Geometry check sheet. Reference: the model listing, model coordinates, mm. Round coordinates to 2 decimals unless told otherwise and drop trailing zeros. Write each loop counter-clockwise with the first axis right and the second up, starting at its lowest first coordinate (ties: lowest second). Pieces come first, ordered by that corner, then holes. Notation, with made-up numbers: (-31, 24) -> (10, 24) arc R18 ccw to (10, 30) -> close; hole circle Ø11 at (65.25, 56.25). An arc over 180 degrees is marked (long way). One line per question, with ' | ' between items.
```python
from build123d import *

# Parameters (mm, degrees)
F1_DEPTH  = 38.1
F2_R      = 9.3756609964
F3_DEPTH  = 50.8
F5_DEPTH  = 76.2
F7_DEPTH  = 76.2
F9_DEPTH  = 76.2
F11_DEPTH = 76.2
F13_DEPTH = 76.2
F14_R     = 1.8366933485
F16_DEPTH = 76.2
F15_R     = 1.8367030573
F17_DEPTH = 76.2


with BuildPart() as f1:
    # F0 (on Front) → F1 (new body)
    with BuildSketch(Plane.XZ):
        Polygon((0, 63.5), (0, 0), (302.4093748547, 0), (302.4093748547, 25.4), align=None)
    extrude(amount=F1_DEPTH)

    # F2 (on face) → F3 (cut)
    with BuildSketch(Plane(origin=(0, 0, 0), x_dir=(0, -1, 0), z_dir=(-1, 0, 0))):
        with Locations((19.05, 31.75)):
            Circle(F2_R)
    extrude(amount=-F3_DEPTH, mode=Mode.SUBTRACT)

    # F4 (on face) → F5 (cut)
    with BuildSketch(Plane.XZ.offset(38.1)):
        with BuildLine():
            Line((269.3568159992, 29.5642309965), (61.5471690917, 55.7457855564))
            add(Edge.make_bspline(
                [(61.5471690917, 55.7457855564), (58.8507788185, 47.0996876999), (48.0888197805, 12.590977334), (174.5673004743, 22.2930190768), (269.3568159992, 29.5642309965)],
                knots=[0, 0, 0, 0, 0.2505482751, 1, 1, 1, 1], degree=3))
        make_face()
    extrude(amount=-F5_DEPTH, mode=Mode.SUBTRACT)

    # F6 (on face) → F7 (cut)
    with BuildSketch(Plane.XZ.offset(38.1)):
        with BuildLine():
            Line((0, 63.5), (0, 49.8412624001))
            Line((0, 49.8412624001), (59.7987414655, 49.8412624001))
            add(Edge.make_bspline(
                [(61.5471690917, 55.7457855564), (60.9299090319, 53.7665131444), (60.3126489722, 51.7872407325), (59.7987414655, 49.8412624001)],
                knots=[0, 0, 0, 0, 0.057355734, 0.057355734, 0.057355734, 0.057355734], degree=3))
            Line((61.5471690917, 55.7457855564), (0, 63.5))
        make_face()
    extrude(amount=-F7_DEPTH, mode=Mode.SUBTRACT)

    # F8 (on face) → F9 (cut)
    with BuildSketch(Plane.XZ.offset(38.1)):
        with BuildLine():
            Line((59.7987414655, 49.8412624001), (52.5512769818, 49.8412624001))
            Line((52.5512769818, 49.8412624001), (59.7987414652, 35.7225287025))
            add(Edge.make_bspline(
                [(59.7987414655, 49.8412624001), (58.4403182232, 44.6974142144), (57.8040351338, 39.7861968724), (59.7987414652, 35.7225287025)],
                knots=[0.057355734, 0.057355734, 0.057355734, 0.057355734, 0.2089654324, 0.2089654324, 0.2089654324, 0.2089654324], degree=3))
        make_face()
    extrude(amount=-F9_DEPTH, mode=Mode.SUBTRACT)

    # F10 (on face) → F11 (cut)
    with BuildSketch(Plane.XZ.offset(38.1)):
        Polygon((302.4093748547, 25.4), (269.3568159992, 29.5642309965), (302.4093748547, 6.536568515), align=None)
    extrude(amount=-F11_DEPTH, mode=Mode.SUBTRACT)

    # F12 (on face) → F13 (cut)
    with BuildSketch(Plane.XZ.offset(38.1)):
        with BuildLine():
            add(Edge.make_bspline(
                [(240.1607868718, 27.3452845776), (249.8366976467, 28.0668616255), (259.596756823, 28.815546311), (269.3568159992, 29.5642309965)],
                knots=[0.9228322548, 0.9228322548, 0.9228322548, 0.9228322548, 1, 1, 1, 1], degree=3))
            Line((240.1607868718, 27.3452845776), (302.4093748547, 6.536568515))
            Line((302.4093748547, 6.536568515), (269.3568159992, 29.5642309965))
        make_face()
    extrude(amount=-F13_DEPTH, mode=Mode.SUBTRACT)

    # F14 (on face) → F16 (cut)
    with BuildSketch(Plane.XZ.offset(38.1)):
        with Locations((6.889551878, 5.4092812352)):
            Circle(F14_R)
    extrude(amount=-F16_DEPTH, mode=Mode.SUBTRACT)

    # F15 (on face) → F17 (cut)
    with BuildSketch(Plane.XZ.offset(38.1)):
        with Locations((292.2985553741, 3.6882217973)):
            Circle(F15_R)
    extrude(amount=-F17_DEPTH, mode=Mode.SUBTRACT)


solid = f1.part
```
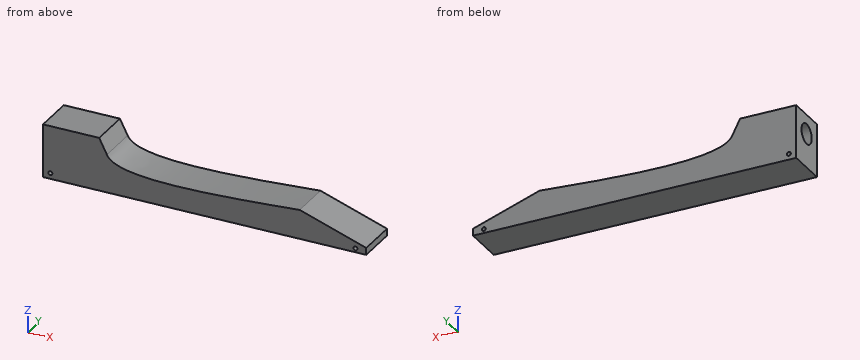
(1) Sectioned sample at B-B on y = -24. Count the separate pieces of the cut face and the enclosed holes in it, then the cut area to 3 significant figures.
Resolved:
separate pieces: 1 | enclosed holes: 2 | area: 7,500 mm2
(2) Sectioned sample at C-C on x = 259.5. Record the cut outline in (y, z).
Resolved:
outline: (-38.1, 0) -> (0, 0) -> (0, 20.88) -> (-38.1, 20.88) -> close
(3) Go/stop test with flat-tipped pins: pin 1 (15 mm diameter, centred on y = -18.5, z = 33.5, fed in from -X); pin 2 (4 mm diameter, centred on y = -19, z = 30.5, fed in from +X). Record where each tip stops, or that it passes through.
Resolved:
pin 1: stops at x = 50.8 | pin 2: stops at x = 68.5
(4) Material ranges on line 1 (X direction, y = -25, z = 3.5); line 2 (X direction, y = -22.5, z = 4); line 3 (Z direction, x = 30, y = -19.05), recorded low to high.
Resolved:
line 1: x = 0 to 290.47, 294.13 to 302.41 | line 2: x = 0 to 5.71, 8.07 to 290.49, 294.11 to 302.41 | line 3: z = 0 to 22.37, 41.13 to 49.84
(5) Sectioned sample at A-A on z = 10. Record the cut outline in (x, y).
Resolved:
outline: (0, -38.1) -> (292.05, -38.1) -> (292.05, 0) -> (0, 0) -> close
